from build123d import *

# Parameters (mm, degrees)
EXTRUDE_THIN1_DEPTH      = 420
EXTRUDE_THIN1_DEPTH_BACK = 420
CUT_EXTRUDE1_DEPTH       = 423.82147533
CUT_EXTRUDE1_DEPTH_BACK  = 423.82147533
SKETCH3_R                = 5


with BuildPart() as part:
    # Sketch1 → Extrude-Thin1 (new, two sides: drawn at the far end of the back side and taken through both)
    with BuildSketch(Plane(origin=(0, 0, 0), x_dir=(0, 0, -1), z_dir=(1, 0, 0)).offset(-EXTRUDE_THIN1_DEPTH_BACK)):
        with BuildLine():
            Line((-23, 35), (-23, -35))
            ThreePointArc((-23, -35), (-20.656854249, -40.656854249), (-15, -43))
            Line((-15, -43), (15, -43))
            ThreePointArc((15, -43), (20.656854249, -40.656854249), (23, -35))
            Line((23, -35), (23, 35))
            ThreePointArc((23, 35), (20.656854249, 40.656854249), (15, 43))
            Line((15, 43), (-15, 43))
            ThreePointArc((-15, 43), (-20.656854249, 40.656854249), (-23, 35))
        make_face()
        with BuildLine():
            Line((-20, 35), (-20, -35))
            ThreePointArc((-20, -35), (-18.535533906, -38.535533906), (-15, -40))
            Line((-15, -40), (15, -40))
            ThreePointArc((15, -40), (18.535533906, -38.535533906), (20, -35))
            Line((20, -35), (20, 35))
            ThreePointArc((20, 35), (18.535533906, 38.535533906), (15, 40))
            Line((15, 40), (-15, 40))
            ThreePointArc((-15, 40), (-18.535533906, 38.535533906), (-20, 35))
        make_face(mode=Mode.SUBTRACT)
    extrude(amount=EXTRUDE_THIN1_DEPTH + EXTRUDE_THIN1_DEPTH_BACK)

    # Sketch3 → Cut-Extrude1 (cut, two sides: drawn at the far end of the back side and taken through both)
    with BuildSketch(Plane(origin=(0, 0, 0), x_dir=(1, 0, 0), z_dir=(0, 1, 0)).offset(-CUT_EXTRUDE1_DEPTH_BACK)):
        with Locations(Location((-387.5, 0, 0), (0, 0, 270))):
            Circle(SKETCH3_R)
        with Locations(Location((-312.5, 0, 0), (0, 0, 270))):
            Circle(SKETCH3_R)
        with Locations(Location((387.5, 0, 0), (0, 0, 90))):
            Circle(SKETCH3_R)
        with Locations(Location((312.5, 0, 0), (0, 0, 90))):
            Circle(SKETCH3_R)
    extrude(amount=CUT_EXTRUDE1_DEPTH + CUT_EXTRUDE1_DEPTH_BACK, mode=Mode.SUBTRACT)


solid = part.part
For this review, take the finished solid that the model builds, in its own axes (mm). A direction names the side the tool comes from. Give positions to 0.01 mm unless a question says otherwise; leave off trailing zeros. Loops run counter-clockwise (first coordinate to the right, second up) from the corner with the lowest first, then second, coordinate; pieces in that order, holes last. Notation, with made-up numbers: (7, -16) - (37, -16) arc R16 ccw to (37, 4) - close; hole circle Ø11 at (6.5, 8). An arc over 180 degrees is marked (long way). Write each question's results on one line, items separated by ' | '.
(1) Draft analysis for pull direction Z (two halves, no side actions). For faces 3 (the flat face through (-6, 40, 0)), 4 (the flat face through (-6, 43, 0)), 5 (the flat face through (-6, 0, -23)), state which applies: +Z half, -Z half, draft (parallel to the pull), parting line (faces both ways), or undercut.
Conclusion:
face 3: undercut | face 4: draft | face 5: -Z half
(2) For pin 1 Ø6 at (x, z) = (387.5, 0) entering from -Y, flat-tipped, find the tip position at first contact; note if it passes through.
Conclusion:
pin 1: through
(3) For faces 1 (the flat face through (-6, 0, 20)), 2 (the flat face through (-420, 3, 21)), list the 3-axis set-ups (+Z, -Z, +X, -X, +Y, -Y) from which the entire face can be reached by the end or side of a thin tool; tool diameter is ignored.
Conclusion:
face 1: +X, -X | face 2: +Z, -Z, -X, +Y, -Y
(4) Take a section at B-B (x = 121.5). Give the boundary of the cut face in (y, z), then the cut area to 3 significant figures.
Conclusion:
outline: (-43, -15) arc R8 ccw to (-35, -23) - (35, -23) arc R8 ccw to (43, -15) - (43, 15) arc R8 ccw to (35, 23) - (-35, 23) arc R8 ccw to (-43, 15) - close; hole (-40, -15) arc R5 ccw to (-35, -20) - (35, -20) arc R5 ccw to (40, -15) - (40, 15) arc R5 ccw to (35, 20) - (-35, 20) arc R5 ccw to (-40, 15) - close | area: 723 mm^2
(5) Take a section at A-A (y = 13). Give the boundary of the cut face in (x, z).
Conclusion:
outline: (-420, -23) - (420, -23) - (420, -20) - (-420, -20) - close; (-420, 20) - (420, 20) - (420, 23) - (-420, 23) - close
(6) For line 1 along X through (y, z) = (41, 0); line 2 along Z through (x, y) = (137, 22.5); line 3 along Y through (x, z) = (-324, -1.5), list the stretches that pass through material, from the lowest coordinate up.
Conclusion:
line 1: -420 to -392.5, -382.5 to -317.5, -307.5 to 307.5, 317.5 to 382.5, 392.5 to 420 | line 2: -23 to -20, 20 to 23 | line 3: -43 to -40, 40 to 43
